Read the model definition and answer for the solid it produces. Units are mm, in the model's axes. A direction names the side the tool comes from. Coordinates: 2 decimals unless noted, no trailing zeros. Order: outer loops, then holes, each group sorted by start corner. A loop starts at its lowest first (then second) coordinate and runs counter-clockwise, first axis right, second up.
```python
from build123d import *

# Parameters (mm, degrees)
SKETCH1_W                = 228.6
SKETCH1_H                = 228.6
BOSS_EXTRUDE1_DEPTH      = 5.08
SKETCH2_W                = 25.4
SKETCH2_H                = 80
CUT_EXTRUDE1_DEPTH       = 5.08
SKETCH3_W                = 5.08
SKETCH3_H                = 12.7
SKETCH3_H_2              = 50.8
CUT_EXTRUDE2_DEPTH       = 5.08
CUT_EXTRUDE4_DEPTH       = 5.08
MIRROR4_COPY_1_DEPTH     = 5.08
CUT_EXTRUDE6_REACH       = 7.08
SKETCH7_W                = 50.8
SKETCH7_H                = 6.35
M3_CLEARANCE_HOLE1_D     = 3.6
M3_CLEARANCE_HOLE1_DEPTH = 5.08
M3_CLEARANCE_HOLE2_D     = 3.6
M3_CLEARANCE_HOLE2_DEPTH = 5.08
SKETCH19_R               = 1.799999956
CUT_EXTRUDE7_DEPTH       = 5.08
MIRROR6_COPY_1_SKETCH_R  = 1.799999956
MIRROR6_COPY_1_DEPTH     = 5.08


with BuildPart() as part:
    # Sketch1 → Boss-Extrude1 (new body)
    with BuildSketch(Plane(origin=(0, 0, 0), x_dir=(1, 0, 0), z_dir=(0, 1, 0))):
        with Locations((114.3, 114.3)):
            Rectangle(SKETCH1_W, SKETCH1_H)
    extrude(amount=BOSS_EXTRUDE1_DEPTH)

    # Sketch2 → Cut-Extrude1 (cut)
    with BuildSketch(Plane(origin=(0, 5.08, 0), x_dir=(1, 0, 0), z_dir=(0, 1, 0))):
        with Locations((12.7, 114.3)):
            Rectangle(SKETCH2_W, SKETCH2_H)
    cut_extrude1 = extrude(amount=-CUT_EXTRUDE1_DEPTH, mode=Mode.SUBTRACT)

    # Mirror1: Cut-Extrude1 across plane
    add(cut_extrude1.mirror(Plane.ZY.offset(-114.3)), mode=Mode.SUBTRACT)

    # Sketch3 → Cut-Extrude2 (cut)
    with BuildSketch(Plane.XZ):
        with Locations((27.94, -171.45)):
            Rectangle(SKETCH3_W, SKETCH3_H)
        with Locations((27.94, -114.3)):
            Rectangle(SKETCH3_W, SKETCH3_H_2)
        with Locations((27.94, -57.15)):
            Rectangle(SKETCH3_W, SKETCH3_H)
    cut_extrude2 = extrude(amount=-CUT_EXTRUDE2_DEPTH, mode=Mode.SUBTRACT)

    # Mirror2: Cut-Extrude2 across plane
    add(cut_extrude2.mirror(Plane.ZY.offset(-114.3)), mode=Mode.SUBTRACT)

    # Sketch5 → Cut-Extrude4 (cut)
    with BuildSketch(Plane.XZ):
        with BuildLine():
            Line((0, -76.2), (0, 0))
            Line((0, 0), (76.2, 0))
            ThreePointArc((76.2, 0), (22.318463274, -22.318463274), (0, -76.2))
        make_face()
    cut_extrude4 = extrude(amount=-CUT_EXTRUDE4_DEPTH, mode=Mode.SUBTRACT)

    # Mirror3: Cut-Extrude4 across plane
    add(cut_extrude4.mirror(Plane.ZY.offset(-114.3)), mode=Mode.SUBTRACT)

    # Mirror4: Cut-Extrude4 across plane
    add(cut_extrude4.mirror(Plane.XY.offset(-114.3)), mode=Mode.SUBTRACT)

    # Mirror4 copy 1 sketch → Mirror4 copy 1 (cut)
    with BuildSketch(Plane(origin=(228.6, 0, -228.6), x_dir=(-1, 0, 0), z_dir=(0, -1, 0))):
        with BuildLine():
            Line((0, -76.2), (0, 0))
            Line((0, 0), (76.2, 0))
            ThreePointArc((76.2, 0), (22.318463274, -22.318463274), (0, -76.2))
        make_face()
    extrude(amount=-MIRROR4_COPY_1_DEPTH, mode=Mode.SUBTRACT)

    # Sketch7 → Cut-Extrude6 (cut, up to next)
    with BuildSketch(Plane(origin=(0, 5.08, 0), x_dir=(1, 0, 0), z_dir=(0, 1, 0)), mode=Mode.PRIVATE) as cut_extrude6_sk1:
        with Locations((114.3, 114.3)):
            Rectangle(SKETCH7_W, SKETCH7_H)
    cut_extrude6_tool1 = extrude(cut_extrude6_sk1.sketch, amount=-CUT_EXTRUDE6_REACH, mode=Mode.PRIVATE) & part.part
    add(cut_extrude6_tool1.solids().sort_by_distance((114.3, 5.08, -114.3))[0], mode=Mode.SUBTRACT)

    # M3 Clearance Hole1
    with Locations(Plane(origin=(0, 5.08, 0), x_dir=(1, 0, 0), z_dir=(0, 1, 0))):
        with Locations((107.41154214, 131.464372429), (107.41154214, 168.964372429), (69.91154214, 131.464372429), (69.91154214, 168.964372429)):
            Hole(M3_CLEARANCE_HOLE1_D / 2, depth=M3_CLEARANCE_HOLE1_DEPTH)

    # M3 Clearance Hole2
    with Locations(Plane(origin=(0, 5.08, 0), x_dir=(1, 0, 0), z_dir=(0, 1, 0))):
        with Locations((72.49651655, 30.046201608), (140.79651655, 30.046201608), (79.19651655, 105.446201608), (133.08651655, 105.446201608)):
            Hole(M3_CLEARANCE_HOLE2_D / 2, depth=M3_CLEARANCE_HOLE2_DEPTH)

    # Sketch19 → Cut-Extrude7 (cut)
    with BuildSketch(Plane.XZ):
        with Locations((200.66, -67.839999956)):
            Circle(SKETCH19_R)
    cut_extrude7 = extrude(amount=-CUT_EXTRUDE7_DEPTH, mode=Mode.SUBTRACT)

    # Mirror5: Cut-Extrude7 across plane
    add(cut_extrude7.mirror(Plane.XY.offset(-114.3)), mode=Mode.SUBTRACT)

    # Mirror6: Cut-Extrude7 across plane
    add(cut_extrude7.mirror(Plane.ZY.offset(-114.3)), mode=Mode.SUBTRACT)

    # Mirror6 copy 1 sketch → Mirror6 copy 1 (cut)
    with BuildSketch(Plane(origin=(228.6, 0, -228.6), x_dir=(-1, 0, 0), z_dir=(0, -1, 0))):
        with Locations((200.66, -67.839999956)):
            Circle(MIRROR6_COPY_1_SKETCH_R)
    extrude(amount=-MIRROR6_COPY_1_DEPTH, mode=Mode.SUBTRACT)


solid = part.part
```
1) Flat-ended cylindrical pins translate along their axes: pin 1 Ø1 at (y, z) = (1, -130) entering from -X; pin 2 Ø3 at (x, z) = (27.94, -67.84) entering from +Y (3 decimals); pin 3 Ø3 at (x, z) = (34, -172.5) entering from -Y; pin 4 Ø3 at (x, y) = (49, 3.5) entering from -Z. Find the tip coordinate at first contact, or state that the pin passes through.
A:
pin 1: stops at x = 30.48
pin 2: passes through
pin 3: stops at y = 0
pin 4: stops at z = -224.14
2) A cutting plane is placed at B-B, the plane z = -150. Determine the outline of the cut face in (x, y), and give its area (3 significant figures).
A:
outline: (25.4, 0) - (203.2, 0) - (203.2, 5.08) - (25.4, 5.08) - close
area: 903 mm2
3) A cutting plane is placed at C-C, the plane z = -40. Determine the outline of the cut face in (x, y), and give its area (3 significant figures).
A:
outline: (9.15, 0) - (219.45, 0) - (219.45, 5.08) - (9.15, 5.08) - close
area: 1,070 mm2
4) Determine the mould class of faces 1 (the flat face through (25.4, 3, -57)), 2 (the flat face through (113, 0, -91)), 3 (the flat face through (28, 3, -88.9)), 4 (the flat face through (114, 3, 0)) for opening direction Z: pulls with the +Z half, pulls with the -Z half, needs draft (parallel to the pull), parting line crosses it, or undercut.
A:
face 1: undercut
face 2: needs draft
face 3: undercut
face 4: pulls with the +Z half
5) Which of the six approach directions +Z, -Z, +X, -X, +Y, -Y give full straight-line access (tool end or side, diameter ignored) to faces 5 (the flat face through (13, 3, -154.3)), 6 (the flat face through (28, 3, -50.8)), 7 (the cylindrical face through (205.012, 2.504, -21.078)), 8 (the flat face through (201, 3, -88.9))?
A:
face 5: -X, +Y, -Y
face 6: +Y, -Y
face 7: +Z, +X, +Y, -Y
face 8: +X, +Y, -Y
6) Straight lines are drawn through the part: line 1 (X direction, y = 1.5, z = -57); line 2 (Z direction, x = 89.5, y = 4.55) (3 decimals); line 3 (Z direction, x = 27.94, y = 3.6). For each, find the intervals that lie inside material, in ascending order.
A:
line 1: x = 2.46 to 25.4, 30.48 to 198.12, 203.2 to 226.14
line 2: z = -228.6 to -117.475, -111.125 to 0
line 3: z = -211.37 to -177.8, -165.1 to -162.56, -158.96 to -139.7, -88.9 to -69.64, -66.04 to -63.5, -50.8 to -17.23
7) A cutting plane is placed at A-A, the plane y = 3.55. State how many separate pieces and enclosed holes the cut face has, and give its area (3 significant figures).
A:
separate pieces: 1
enclosed holes: 17
area: 42,000 mm2
